from build123d import *

# Parameters (mm, degrees)
F0_W     = 100
F0_H     = 50
F1_DEPTH = 80
F2_W     = 50
F2_H     = 50
F3_DEPTH = 50
F4_SIZE  = 20
F5_R     = 7.5
F6_DEPTH = 30


with BuildPart() as f1:
    # F0 (on Top) → F1 (new body)
    with BuildSketch(Plane.XY):
        with Locations((5.763268, -25.05821)):
            Rectangle(F0_W, F0_H)
    extrude(amount=F1_DEPTH)

    # F2 (on face) → F3 (cut, through all)
    with BuildSketch(Plane.XZ.offset(50.05821)):
        with Locations((30.763268, 55)):
            Rectangle(F2_W, F2_H)
    extrude(amount=-F3_DEPTH, mode=Mode.SUBTRACT)

    # F4
    f4_edges = [f1.edges().sort_by_distance(p)[0] for p in [
        (-44.236732, -25.05821, 80),
    ]]
    chamfer(f4_edges, length=F4_SIZE)

    # F5 (on face) → F6 (cut, through all)
    with BuildSketch(Plane.XY.offset(30)):
        with Locations((30.763268, -25.05821)):
            Circle(F5_R)
    extrude(amount=-F6_DEPTH, mode=Mode.SUBTRACT)


solid = f1.part
Read the model definition and answer for the solid it produces. Units are mm, in the model's axes. A direction names the side the tool comes from. Coordinates: 2 decimals unless noted, no trailing zeros. Order: outer loops, then holes, each group sorted by start corner. A loop starts at its lowest first (then second) coordinate and runs counter-clockwise, first axis right, second up. Notation, with made-up numbers: M 58,71.5 L 71,71.5 A26 ccw 71,91.5 Z; hole C -11.5,-24 d9. An arc over 180 degrees is marked long. Put each result on its own line as item: value. Start each with the question number.
Item 1: The mould has two halves that part along X. Classify faces 1 (the face through (37.69, -27.93, 15.21)), 2 (the face through (-9, -25, 80)), 3 (the face through (-34.097, -25.408, 70.14)), 4 (the face through (5.763, -25, 55)): +X half, -X half, draft (parallel to the pull), parting line (faces both ways), or undercut.
Item 2: Section C-C, the plane y = -10 is taken. Determine the outline of the cut face in (x, z), plus the area to 3 significant figures.
Item 3: Consider probe 1 along Z at (x, y) = (23.5, -36.5); probe 2 along X at (y, z) = (-15, 59); probe 3 along X at (y, z) = (-30.5, 16.5). Determine where each line is inside the solid, lowest interval first. Write a range as [from, to].
Item 4: Given pin 1 Ø1.5 at (x, y) = (43.5, -35.5) entering from -Z; pin 2 Ø12 at (x, y) = (30.76, -25.06) entering from +Z, each flat-ended and moving along its own axis, determine where each tip first touches the part or whether it passes through.
Item 5: Section D-D, the plane z = 46 is taken. Determine the outline of the cut face in (x, y).
Item 6: Section A-A, the plane y = -19.5 is taken. Determine the outline of the cut face in (x, z), plus the area to 3 significant figures.
Item 7: Section B-B, the plane x = 28 is taken. Determine the outline of the cut face in (y, z), plus the area to 3 significant figures.
Item 8: For faces 5 (the face through (25, -31, 30)), 6 (the face through (-44.237, -25, 30)), determine the directions among +Z, -Z, +X, -X, +Y, -Y from which every point of the face is accessible in a straight line to the end or side of a thin tool.
Computed:
1. face 1: undercut
1. face 2: draft
1. face 3: -X half
1. face 4: +X half
2. outline: M -44.24,0 L 55.76,0 L 55.76,30 L 5.76,30 L 5.76,80 L -24.24,80 L -44.24,60 Z
2. area: 5,300 mm2
3. probe 1: z = [0, 30]
3. probe 2: x = [-44.24, 5.76]
3. probe 3: x = [-44.24, 25.6], [35.92, 55.76]
4. pin 1: stops at z = 0
4. pin 2: passes through
5. outline: M -44.24,-50.06 L 5.76,-50.06 L 5.76,-0.06 L -44.24,-0.06 Z
6. outline: M -44.24,0 L 25.73,0 L 25.73,30 L 5.76,30 L 5.76,80 L -24.24,80 L -44.24,60 Z; M 35.8,0 L 55.76,0 L 55.76,30 L 35.8,30 Z
6. area: 5,000 mm2
7. outline: M -50.06,0 L -32.03,0 L -32.03,30 L -50.06,30 Z; M -18.09,0 L -0.06,0 L -0.06,30 L -18.09,30 Z
7. area: 1,080 mm2
8. face 5: +Z, +X, +Y, -Y
8. face 6: +Z, -Z, -X, +Y, -Y
